Part model, mm, in its own coordinate system. A direction names the side the tool comes from. Coordinates: 2 decimals unless noted, no trailing zeros. Loops run counter-clockwise (first coordinate to the right, second up) from the corner with the lowest first, then second, coordinate; pieces in that order, holes last. Notation, with made-up numbers: (-17, -0.75) - (35, -0.75) arc R26 cw to (35, 29.25) - close; hole circle Ø3 at (-15, -12.5). An arc over 180 degrees is marked (long way). Use a Markdown table: item, result. Add a question column.
1. Band-saw the part on B-B, the plane x = 27.5. Give the cut face in (y, z) (3 decimals), plus the area to 3 significant figures.
2. Wall check: probe 1 along Z at (x, y) = (5.5, -1) (3 decimals); probe 2 along X at (y, z) = (-7.25, -9.5) (3 decimals); probe 3 along X at (y, z) = (-7, -10) (3 decimals). Give the ranges that are in metal, low to high. Write a range as [from, to].
3. Drop flat-ended pins along their axis: pin 1 (2 mm diameter, centred on x = 31, z = 15.5, fed in from +Y); pin 2 (16 mm diameter, centred on x = -18.5, z = 2, fed in from +Y). Give the stop position or say it passes through.
4. Band-saw the part on A-A, the plane y = -7. Count the separate pieces of the cut face and the enclosed holes in it, plus the area to 3 significant figures.
5. Pull direction Z, two halves, no side cores. Call faces 1 (the flat face through (-1, -6, 22.225)), 2 (the cylindrical face through (-38.2, -0.7, 16)), 3 (the cylindrical face through (-38.3, -0.7, -16)), 4 (the flat face through (53.975, -6, 0)): pulls with the +Z half, pulls with the -Z half, needs draft (parallel to the pull), parting line crosses it, or undercut.
6. Band-saw the part on C-C, the plane x = 39. Give the cut face in (y, z) (3 decimals).
7. 3-axis set-ups, long thin cutter, end or side, ignore diameter. For faces 5 (the cylindrical face through (-48.75, -6.44, 6.61)), 6 (the cylindrical face through (38.3, -0.7, 16)): which of +Z, -Z, +X, -X, +Y, -Y reach the whole face in a straight line?
from build123d import *

# Parameters (mm, degrees)
SKETCH1_W             = 107.95
SKETCH1_H             = 44.45
BOSS_EXTRUDE1_DEPTH   = 12.7
CUT_EXTRUDE1_DEPTH    = 1.397
M5X0_8_TAPPED_HOLE1_D = 4.2


with BuildPart() as part:
    # Sketch1 → Boss-Extrude1 (new body)
    with BuildSketch(Plane(origin=(0, 0, 0), x_dir=(1, 0, 0), z_dir=(0, 1, 0))):
        Rectangle(SKETCH1_W, SKETCH1_H)
    extrude(amount=-BOSS_EXTRUDE1_DEPTH)

    # Sketch2 → Cut-Extrude1 (cut)
    with BuildSketch(Plane(origin=(0, 0, 0), x_dir=(1, 0, 0), z_dir=(0, 1, 0))):
        with BuildLine():
            Line((41.402, 12.827), (41.402, -12.827))
            ThreePointArc((41.402, -12.827), (38.227, -16.002), (35.052, -12.827))
            Line((35.052, -12.827), (-35.052, -12.827))
            ThreePointArc((-35.052, -12.827), (-38.227, -16.002), (-41.402, -12.827))
            Line((-41.402, -12.827), (-41.402, 12.827))
            ThreePointArc((-41.402, 12.827), (-38.227, 16.002), (-35.052, 12.827))
            Line((-35.052, 12.827), (35.052, 12.827))
            ThreePointArc((35.052, 12.827), (38.227, 16.002), (41.402, 12.827))
        make_face()
    extrude(amount=-CUT_EXTRUDE1_DEPTH, mode=Mode.SUBTRACT)

    # M5x0.8 Tapped Hole1 (through all)
    with Locations(Plane(origin=(0, 0, 0), x_dir=(1, 0, 0), z_dir=(0, 1, 0))):
        with Locations((-47.625, 8.382), (-47.625, 2.794), (-47.625, -2.794), (-47.625, -8.382), (47.625, -8.382), (47.625, -2.794), (47.625, 2.794), (47.625, 8.382)):
            Hole(M5X0_8_TAPPED_HOLE1_D / 2)


solid = part.part
Geometry check:
| question | item | result |
|---|---|---|
| 1 | outline | (-12.7, -22.225) - (0, -22.225) - (0, -12.827) - (-1.397, -12.827) - (-1.397, 12.827) - (0, 12.827) - (0, 22.225) - (-12.7, 22.225) - close |
| 1 | area | 529 mm^2 |
| 2 | probe 1 | z = [-22.225, -12.827], [12.827, 22.225] |
| 2 | probe 2 | x = [-53.975, -49.403], [-45.847, 45.847], [49.403, 53.975] |
| 2 | probe 3 | x = [-53.975, -48.964], [-46.286, 46.286], [48.964, 53.975] |
| 3 | pin 1 | stops at y = 0 |
| 3 | pin 2 | stops at y = -1.4 |
| 4 | separate pieces | 1 |
| 4 | enclosed holes | 8 |
| 4 | area | 4,690 mm^2 |
| 5 | face 1 | pulls with the +Z half |
| 5 | face 2 | undercut |
| 5 | face 3 | undercut |
| 5 | face 4 | needs draft |
| 6 | outline | (-12.7, -22.225) - (0, -22.225) - (0, -15.906) - (-1.397, -15.906) - (-1.397, 15.906) - (0, 15.906) - (0, 22.225) - (-12.7, 22.225) - close |
| 7 | face 5 | +Y, -Y |
| 7 | face 6 | +Y |
